Geometry: final body of the model. Coordinates: model frame, mm. Face numbers are marked on the shaded views. A direction names the side the tool comes from. Give positions to 0.01 mm unless a question says otherwise; leave off trailing zeros. Order: outer loops, then holes, each group sorted by start corner. A loop starts at its lowest first (then second) coordinate and runs counter-clockwise, first axis right, second up. Notation, with made-up numbers: (-13.5, 86.25) - (-0.5, 86.25) arc R23 ccw to (-0.5, 111.25) - close; hole circle Ø8 at (-35.5, 66.25). An arc over 180 degrees is marked (long way). Put each result on its own line as item: value. Start each with the question number.
1. First-contact query: P1, Ø5, axis at y = 4.5, z = -27, coming from the -X side; P2, Ø1.5, axis at y = 13, z = -29.5, coming from the +X side. Flat tips, straight axial feed; report the tip coordinate or a pass-through.
2. Ray query, line 1 along X through (y, z) = (9, 13); line 2 along Z through (x, y) = (-29.5, 1.75); line 3 along X through (y, z) = (9.5, -24). Return the intervals inside material, ascending. Write a range as from..to.
3. Section A-A on y = 9. Return the cut outline in (x, z).
4. Section B-B on z = 26. Return the cut outline in (x, y).
5. Section D-D on x = -19.5. Return the cut outline in (y, z), plus the area to 3 significant figures.
6. Set-up query: the marked faces 5 and 6. Return all of +Z, -Z, +X, -X, +Y, -Y with unobstructed straight access to the full face (end or side cutting, diameter ignored); none if empty.
7. Mould query, pull axis X, two halves, no side actions, for the marked faces 1, 2, 3 and 4. Classes: pulls with the +X half, pulls with the -X half, needs draft (parallel to the pull), parting line crosses it, or undercut.
8. Section C-C on y = 16.75. Return the cut outline in (x, z), plus the area to 3 significant figures.
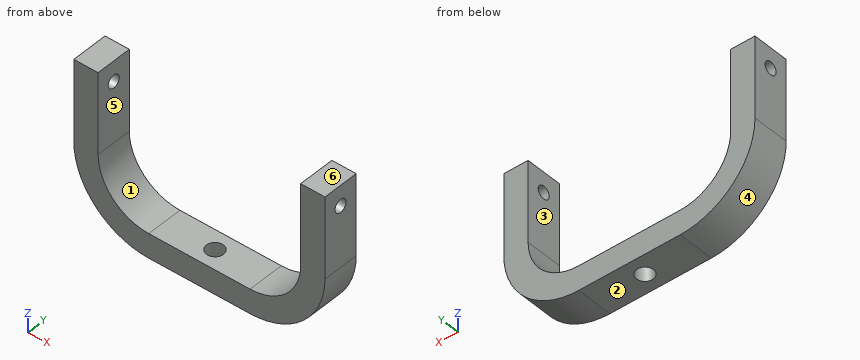
from build123d import *

# Parameters (mm, degrees)
BOSS_EXTRUDE1_DEPTH     = 18
SKETCH2_R               = 3.2
CUT_EXTRUDE1_DEPTH      = 150
CUT_EXTRUDE1_DEPTH_BACK = 40
SKETCH3_R               = 4.2
CUT_EXTRUDE2_DEPTH      = 40


with BuildPart() as part:
    # Sketch1 → Boss-Extrude1 (new body)
    with BuildSketch(Plane(origin=(0, 0, 0), x_dir=(1, 0, 0), z_dir=(0, 1, 0))):
        with BuildLine():
            Line((-70.033707865, -37.921348315), (-58.033707865, -37.921348315))
            Line((-58.033707865, -37.921348315), (-58.033707865, 2.078651685))
            ThreePointArc((-58.033707865, 2.078651685), (-50.711377395, 19.756321215), (-33.033707865, 27.078651685))
            Line((-33.033707865, 27.078651685), (-8.033707865, 27.078651685))
            Line((-8.033707865, 27.078651685), (-8.033707865, 39.078651685))
            Line((-8.033707865, 39.078651685), (-33.033707865, 39.078651685))
            ThreePointArc((-33.033707865, 39.078651685), (-59.196658769, 28.241602589), (-70.033707865, 2.078651685))
            Line((-70.033707865, 2.078651685), (-70.033707865, -37.921348315))
        make_face()
    boss_extrude1 = extrude(amount=BOSS_EXTRUDE1_DEPTH)

    # Mirror1: Boss-Extrude1 across plane
    add(boss_extrude1.mirror(Plane(origin=(-8.033707865, 18, -39.078651685), x_dir=(0, 0, 1), z_dir=(-1, 0, 0))))

    # Sketch2 → Cut-Extrude1 (cut, two sides)
    with BuildSketch(Plane(origin=(-58.033707865, 0, 0), x_dir=(0, 0, -1), z_dir=(1, 0, 0))) as cut_extrude1_sk:
        with Locations((-27.921348315, 9)):
            Circle(SKETCH2_R)
    extrude(amount=CUT_EXTRUDE1_DEPTH, mode=Mode.SUBTRACT)
    extrude(cut_extrude1_sk.sketch, amount=-CUT_EXTRUDE1_DEPTH_BACK, mode=Mode.SUBTRACT)

    # Sketch3 → Cut-Extrude2 (cut)
    with BuildSketch(Plane.XY.offset(-27.078651685)):
        with Locations((-8.033707865, 9)):
            Circle(SKETCH3_R)
    extrude(amount=-CUT_EXTRUDE2_DEPTH, mode=Mode.SUBTRACT)


solid = part.part
Resolved:
1. P1: x = -62.47
1. P2: x = 42.61
2. line 1: -70.03..-58.03, 41.97..53.97
2. line 2: -39.08..-27.08
2. line 3: -62.84..-45.05, 28.99..46.77
3. outline: (-70.03, -2.08) arc R37 ccw to (-33.03, -39.08) - (-12.23, -39.08) - (-12.23, -27.08) - (-33.03, -27.08) arc R25 cw to (-58.03, -2.08) - (-58.03, 24.72) - (-70.03, 24.72) - close; (-70.03, 31.12) - (-58.03, 31.12) - (-58.03, 37.92) - (-70.03, 37.92) - close; (-3.83, -39.08) - (16.97, -39.08) arc R37 ccw to (53.97, -2.08) - (53.97, 24.72) - (41.97, 24.72) - (41.97, -2.08) arc R25 cw to (16.97, -27.08) - (-3.83, -27.08) - close; (41.97, 31.12) - (53.97, 31.12) - (53.97, 37.92) - (41.97, 37.92) - close
4. outline: (-70.03, 0) - (-58.03, 0) - (-58.03, 6.44) - (-70.03, 6.44) - close; (-70.03, 11.56) - (-58.03, 11.56) - (-58.03, 18) - (-70.03, 18) - close; (41.97, 0) - (53.97, 0) - (53.97, 6.44) - (41.97, 6.44) - close; (41.97, 11.56) - (53.97, 11.56) - (53.97, 18) - (41.97, 18) - close
5. outline: (0, -39.08) - (18, -39.08) - (18, -27.08) - (0, -27.08) - close
5. area: 216 mm^2
6. face 5: +Z, +Y, -Y
6. face 6: +Z, +X, -X, +Y, -Y
7. face 1: undercut
7. face 2: needs draft
7. face 3: undercut
7. face 4: pulls with the -X half
8. outline: (-70.03, -2.08) arc R37 ccw to (-33.03, -39.08) - (16.97, -39.08) arc R37 ccw to (53.97, -2.08) - (53.97, 37.92) - (41.97, 37.92) - (41.97, -2.08) arc R25 cw to (16.97, -27.08) - (-33.03, -27.08) arc R25 cw to (-58.03, -2.08) - (-58.03, 37.92) - (-70.03, 37.92) - close
8. area: 2,730 mm^2
